The model under review builds one solid part; all positions refer to its coordinate system, in mm. A direction names the side the tool comes from. Round coordinates to 2 decimals unless told otherwise and drop trailing zeros. Write each loop counter-clockwise with the first axis right and the second up, starting at its lowest first coordinate (ties: lowest second). Pieces come first, ordered by that corner, then holes. Notation, with made-up numbers: (11.25, 46.25) -> (36.25, 46.25) arc R18 cw to (36.25, 65.25) -> close; hole circle Ø9 at (-35.5, -16). An arc over 180 degrees is marked (long way). Use CSV: the item, a comma, the result in double quotes. Start each with the question number.
1) Take a section at A-A, the plane x = 0. Give the boundary of the cut face in (y, z).
2) Wall thickness on probe 1 along Z at (x, y) = (-1.75, 4) (3 decimals); probe 2 along Y at (x, z) = (4.75, -12.5); probe 3 along Z at (x, y) = (-1.25, 2.5): over which ranges is each line inside the solid? List them lowest first. Write a range as [from, to].
3) Take a section at C-C, the plane y = 1.5. Give the boundary of the cut face in (x, z) (3 decimals).
4) Mouldability with a two-part tool opening along Z and no side actions: class faces 4 (the face through (0, -1, -3)), 5 (the face through (-0.02, 2.94, -2.65)), 6 (the face through (0.66, -0.493, 14.985)) as released by +Z, released by -Z, zero draft, split by the parting line, or undercut.
5) For pin 1 Ø0.6 at (y, z) = (3, 2) entering from +X; pin 2 Ø1.5 at (x, y) = (2.5, 5) entering from +Z; pin 3 Ø2 at (y, z) = (1.5, -3.5) entering from -X, all flat-tipped, find the tip position at first contact; note any pin that passes through.
6) Machinability: for faces 1 (the face through (-2.65, 2.94, 0.02)), 2 (the face through (13.4, 0, 0.1)), 3 (the face through (-2, 7, 2)), which of the approach directions +Z, -Z, +X, -X, +Y, -Y give a long, thin tool a straight path to every point of the face, cutting with its end or side? Answer none if there is none.
from build123d import *

# Parameters (mm, degrees)
SKETCH1_R           = 13
BOSS_EXTRUDE1_DEPTH = 7
SKETCH3_R           = 15
BOSS_EXTRUDE2_DEPTH = 1
SKETCH4_W           = 2.29
SKETCH4_H           = 2.29
CUT_EXTRUDE1_DEPTH  = 23.671568098
FILLET1_R           = 0.5


with BuildPart() as part:
    # Sketch1 → Boss-Extrude1 (new body)
    with BuildSketch(Plane(origin=(0, 0, 0), x_dir=(1, 0, 0), z_dir=(0, 1, 0))):
        with Locations(Location((0, 0, 0), (0, 0, 270))):
            Circle(SKETCH1_R)
    extrude(amount=BOSS_EXTRUDE1_DEPTH)

    # Sketch2 → Cut-Revolve1 (revolve, cut)
    with BuildSketch(Plane(origin=(0, 0, 0), x_dir=(0, 0, -1), z_dir=(1, 0, 0)), mode=Mode.PRIVATE) as cut_revolve1_sk:
        Polygon((-13, 0), (-10.907887029, 7), (-13, 7), align=None)
    revolve(cut_revolve1_sk.sketch.rotate(Axis((0, 0, 0), (0, 1, 0)), 180), axis=Axis((0, 0, 0), (0, 1, 0)), mode=Mode.SUBTRACT)

    # Sketch3 → Boss-Extrude2 (add)
    with BuildSketch(Plane(origin=(0, 0, 0), x_dir=(-1, 0, 0), z_dir=(0, -1, 0))):
        with Locations(Location((0, 0, 0), (0, 0, 90))):
            Circle(SKETCH3_R)
    extrude(amount=BOSS_EXTRUDE2_DEPTH)

    # Sketch4 → Cut-Extrude1 (cut, through all)
    with BuildSketch(Plane.XZ.offset(1)):
        Rectangle(SKETCH4_W, SKETCH4_H)
        with BuildLine():
            Line((-2.389869243, -1.145), (-1.145, -1.145))
            Line((-1.145, -1.145), (-1.145, 1.145))
            Line((-1.145, 1.145), (-2.389869243, 1.145))
            ThreePointArc((-2.389869243, 1.145), (-2.65, 0), (-2.389869243, -1.145))
        make_face()
        with BuildLine():
            Line((-1.145, 1.145), (1.145, 1.145))
            Line((1.145, 1.145), (1.145, 2.389869243))
            ThreePointArc((1.145, 2.389869243), (0, 2.65), (-1.145, 2.389869243))
            Line((-1.145, 2.389869243), (-1.145, 1.145))
        make_face()
        with BuildLine():
            Line((1.145, 1.145), (1.145, -1.145))
            Line((1.145, -1.145), (2.389869243, -1.145))
            ThreePointArc((2.389869243, -1.145), (2.584149134, -0.587088795), (2.65, 0))
            ThreePointArc((2.65, 0), (2.584149134, 0.587088795), (2.389869243, 1.145))
            Line((2.389869243, 1.145), (1.145, 1.145))
        make_face()
        with BuildLine():
            ThreePointArc((-1.145, -2.389869243), (0, -2.65), (1.145, -2.389869243))
            Line((1.145, -2.389869243), (1.145, -1.145))
            Line((1.145, -1.145), (-1.145, -1.145))
            Line((-1.145, -1.145), (-1.145, -2.389869243))
        make_face()
    extrude(amount=-CUT_EXTRUDE1_DEPTH, mode=Mode.SUBTRACT)

    # Fillet1
    fillet1_edges = [part.edges().sort_by_distance(p)[0] for p in [
        (-1.145, 3, 1.145),
        (1.145, 3, 1.145),
        (1.145, 3, -1.145),
        (-1.145, 3, -1.145),
    ]]
    fillet(fillet1_edges, radius=FILLET1_R)


solid = part.part
Values found:
1,outline,"(-1, -15) -> (0, -15) -> (0, -13) -> (7, -10.91) -> (7, -2.65) -> (-1, -2.65) -> close; (-1, 2.65) -> (7, 2.65) -> (7, 10.91) -> (0, 13) -> (0, 15) -> (-1, 15) -> close"
2,probe 1,"[-11.674, -1.145], [1.145, 11.674]"
2,probe 2,"[-1, 0]"
2,probe 3,"[-12.19, -1.34], [1.34, 12.19]"
3,outline,"circle Ø25.103 at (0, 0); hole (-2.39, -1.145) -> (-1.645, -1.145) arc R0.5 cw to (-1.145, -1.645) -> (-1.145, -2.39) arc R2.65 ccw to (1.145, -2.39) -> (1.145, -1.645) arc R0.5 cw to (1.645, -1.145) -> (2.39, -1.145) arc R2.65 ccw to (2.39, 1.145) -> (1.645, 1.145) arc R0.5 cw to (1.145, 1.645) -> (1.145, 2.39) arc R2.65 ccw to (-1.145, 2.39) -> (-1.145, 1.645) arc R0.5 cw to (-1.645, 1.145) -> (-2.39, 1.145) arc R2.65 ccw to start"
4,face 4,"zero draft"
4,face 5,"undercut"
4,face 6,"split by the parting line"
5,pin 1,"x = 12.04"
5,pin 2,"z = 11.51"
5,pin 3,"x = -12.46"
6,face 1,"+Y, -Y"
6,face 2,"+Y"
6,face 3,"+Z, -Z, +X, -X, +Y"
